Work out the finished part from the listing and answer in its coordinate system (mm). Face numbers are marked on the shaded views. A direction names the side the tool comes from. Give positions to 0.01 mm unless a question says otherwise; leave off trailing zeros. Order: outer loops, then holes, each group sorted by start corner. A loop starts at its lowest first (then second) coordinate and runs counter-clockwise, first axis right, second up. Notation, with made-up numbers: (-26, -30.5) - (26, -30.5) arc R32 cw to (26, 3.5) - close; hole circle Ø11 at (58, -38.5). An arc over 180 degrees is marked (long way). Write each question's results on one line, items separated by ' | '.
from build123d import *

# Parameters (mm, degrees)
F1_DEPTH        = 25
F3_START        = -0.65
F2_R            = 4.3
F3_DEPTH        = 2.15
F3_COPIES_COUNT = 3
F6_R            = 33.7024135389
F7_DEPTH        = 2
F9_DEPTH        = 21


# Not quite as in the source:
# - a pattern or mirror of a feature is missing from the dataset's text; its kind, count and spacing are read off the source's solid


with BuildPart() as f1:
    # F0 (on Top) → F1 (new body)
    with BuildSketch(Plane.XY):
        with BuildLine():
            ThreePointArc((7.6794919243, -4), (19.8038475773, 3), (19.8038475773, 17))
            Line((19.8038475773, 17), (12.124355653, 30.3012701892))
            ThreePointArc((12.124355653, 30.3012701892), (0, 37.3012701892), (-12.124355653, 30.3012701892))
            Line((-12.124355653, 30.3012701892), (-19.8038475773, 17))
            ThreePointArc((-19.8038475773, 17), (-19.8038475773, 3), (-7.6794919243, -4))
            Line((-7.6794919243, -4), (0, -4))
            Line((0, -4), (7.6794919243, -4))
        make_face()
        with BuildLine():
            Line((7.6794919243, 0), (0, 0))
            Line((0, 0), (-7.6794919243, 0))
            ThreePointArc((-7.6794919243, 0), (-16.3397459622, 5), (-16.3397459622, 15))
            Line((-16.3397459622, 15), (-8.6602540378, 28.3012701892))
            ThreePointArc((-8.6602540378, 28.3012701892), (0, 33.3012701892), (8.6602540378, 28.3012701892))
            Line((8.6602540378, 28.3012701892), (16.3397459622, 15))
            ThreePointArc((16.3397459622, 15), (16.3397459622, 5), (7.6794919243, 0))
        make_face(mode=Mode.SUBTRACT)
    extrude(amount=F1_DEPTH)

    # F2 (on face) → F3 (cut)
    with BuildSketch(Plane(origin=(-22.2141016151, 12.8253175473, 0), x_dir=(-0.5, -0.8660254038, 0), z_dir=(-0.8660254038, 0.5, 0)).offset(F3_START)):
        with Locations((-12.5, 12.5)):
            Circle(F2_R)
    f3 = extrude(amount=-F3_DEPTH, mode=Mode.SUBTRACT)

    # F3_copies: F3 ×3 about axis
    f3_copies_axis = Axis((0, 14.433757, 0), (0, 0, 1))
    for i in range(1, F3_COPIES_COUNT):
        add(f3.rotate(f3_copies_axis, i * 360 / F3_COPIES_COUNT), mode=Mode.SUBTRACT)

    # F6 (on face) → F7 (cut)
    with BuildSketch(Plane.XY.offset(25)):
        with Locations((0, 15.2027085423)):
            Circle(F6_R)
    extrude(amount=-F7_DEPTH, mode=Mode.SUBTRACT)

    # F8 (on face) → F9 (cut)
    with BuildSketch(Plane.XY.offset(23)):
        with BuildLine():
            Line((-12.124355653, 30.3012701892), (-19.8038475773, 17))
            ThreePointArc((-19.8038475773, 17), (-19.8038475773, 3), (-7.6794919243, -4))
            Line((-7.6794919243, -4), (7.6794919243, -4))
            ThreePointArc((7.6794919243, -4), (19.8038475773, 3), (19.8038475773, 17))
            Line((19.8038475773, 17), (12.124355653, 30.3012701892))
            ThreePointArc((12.124355653, 30.3012701892), (0, 37.3012701892), (-12.124355653, 30.3012701892))
        make_face()
        with BuildLine():
            ThreePointArc((-11.5181378703, 29.9512701892), (0, 36.6012701892), (11.5181378703, 29.9512701892))
            Line((11.5181378703, 29.9512701892), (19.1976297946, 16.65))
            ThreePointArc((19.1976297946, 16.65), (19.1976297946, 3.35), (7.6794919243, -3.3))
            Line((7.6794919243, -3.3), (-7.6794919243, -3.3))
            ThreePointArc((-7.6794919243, -3.3), (-19.1976297946, 3.35), (-19.1976297946, 16.65))
            Line((-19.1976297946, 16.65), (-11.5181378703, 29.9512701892))
        make_face(mode=Mode.SUBTRACT)
    extrude(amount=-F9_DEPTH, mode=Mode.SUBTRACT)


solid = f1.part
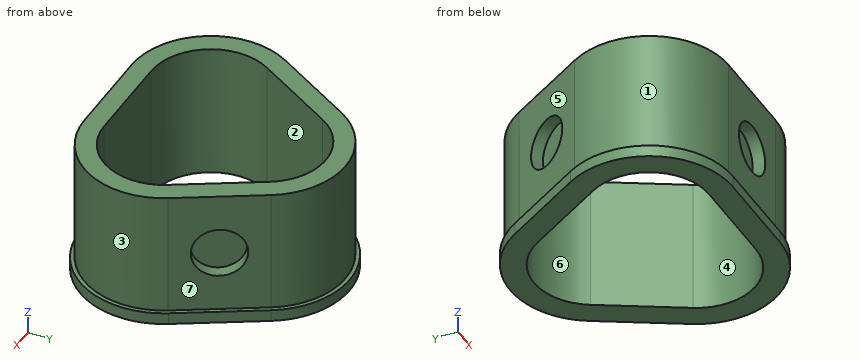
1. A cutting plane is placed at C-C, the plane y = 2. Write down the section's boundary in (x, z).
Answer list:
outline: (-19.17, 0) - (-13.68, 0) - (-13.68, 23) - (-18.3, 23) - (-18.3, 2) - (-19.17, 2) - close; (13.68, 0) - (19.17, 0) - (19.17, 2) - (18.3, 2) - (18.3, 23) - (13.68, 23) - close
2. A cutting plane is placed at D-D, the plane x = 18.5. Write down the section's boundary in (y, z).
Answer list:
outline: (1.12, 0) - (19.26, 0) - (19.26, 2) - (17.86, 2) - (17.86, 23) - (2.27, 23) - (2.27, 2) - (1.12, 2) - close
3. A tool of negligible diameter and unlimited length cuts with its end or side. For the marked faces 1, 2 and 3, from which of +Z, -Z, +X, -X, +Y, -Y can it reach the whole face along a straight path? Write none if from no direction.
Answer list:
face 1: +Z, -X | face 2: +Z, -Z | face 3: +Z, +X
4. A cutting plane is placed at A-A, the plane x = 0. Write down the section's boundary in (y, z), then the cut area to 3 significant figures.
Answer list:
outline: (-4, 0) - (0, 0) - (0, 23) - (-3.3, 23) - (-3.3, 16.8) - (-1.2, 16.8) - (-1.2, 8.2) - (-3.3, 8.2) - (-3.3, 2) - (-4, 2) - close; (33.3, 0) - (37.3, 0) - (37.3, 2) - (36.6, 2) - (36.6, 23) - (33.3, 23) - close | area: 137 mm^2
5. Straight lines are drawn through the part: line 1 (Z direction, x = 0, y = -2.75); line 2 (X direction, y = 10, z = 19.25); line 3 (Y direction, x = -3, z = 2.5). For each, find the intervals that lie inside material, in ascending order. Write a range as [from, to].
Answer list:
line 1: [0, 8.2], [16.8, 23] | line 2: [-20.98, -17.68], [17.68, 20.98] | line 3: [-3.3, 0], [32.84, 36.26]
6. Determine the mould class of the marked faces 4, 5, 6 and 7 for opening direction X: +X half, -X half, draft (parallel to the pull), parting line (faces both ways), or undercut.
Answer list:
face 4: undercut | face 5: -X half | face 6: undercut | face 7: +X half
7. A cutting plane is placed at B-B, the plane z = 2.75. Write down the section's boundary in (x, y).
Answer list:
outline: (-19.2, 16.65) arc R13.3 ccw to (-7.68, -3.3) - (7.68, -3.3) arc R13.3 ccw to (19.2, 16.65) - (11.52, 29.95) arc R13.3 ccw to (-11.52, 29.95) - close; hole (-16.34, 15) arc R10 ccw to (-7.68, 0) - (7.68, 0) arc R10 ccw to (16.34, 15) - (8.66, 28.3) arc R10 ccw to (-8.66, 28.3) - close
8. Given P1, Ø12.5, axis at x = 3.5, z = 8.5, coming from the +Y side; P2, Ø7, axis at x = 1.5, z = 14.5, coming from the -Y side; P3, Ø8, axis at y = 10.5, z = 8.5, coming from the +X side, each flat-ended and moving along its own axis, determine where each tip first touches the part or whether it passes through.
Answer list:
P1: y = 36.6 | P2: y = -3.3 | P3: x = 20.98
